Design review of the part shown in the three views and the two pictorial views. Dimensions are in mm from the part's minimum x, y and z. Coordinates: 2 decimals unless noted, no trailing zeros. Write each loop counter-clockwise with the first axis right and the second up, starting at its lowest first coordinate (ties: lowest second). Pieces come first, ordered by that corner, then holes. Notation, with made-up numbers: M -4.75,-28.75 L 5.25,-28.75 A13 cw 5.25,-14.75 Z; hole C 41.5,-19.5 d7. An arc over 180 degrees is marked long. One line per question, with ' | ' between items.
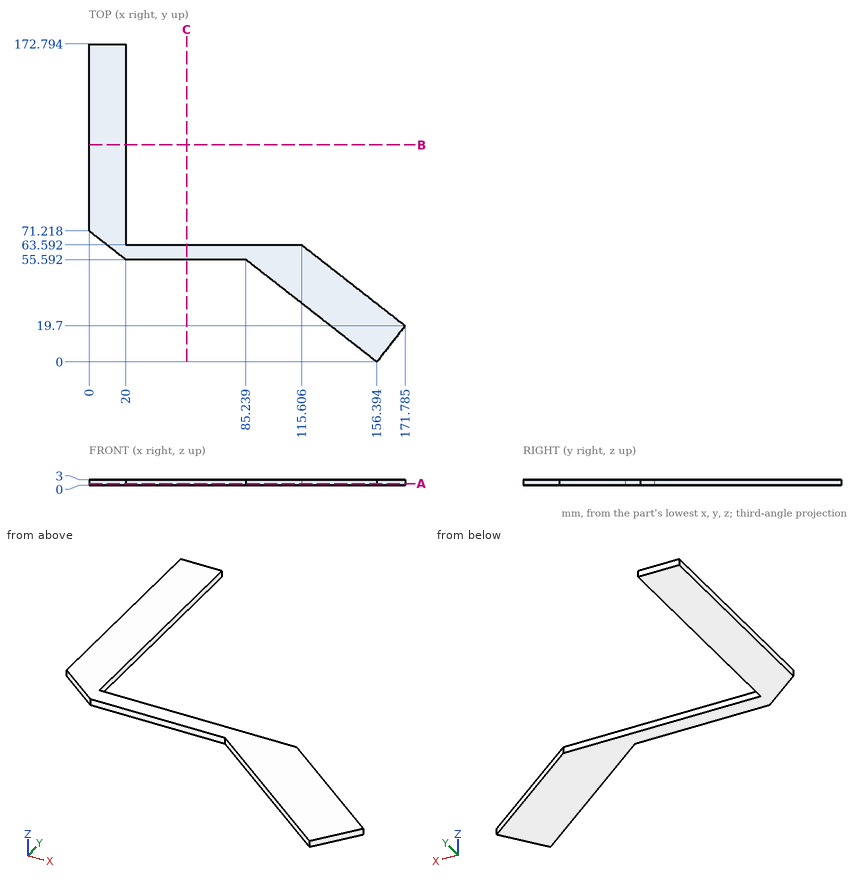
1. Take a section at C-C on x = 53. State the section outline as (y, z) points.
Computed values:
outline: M 55.59,0 L 63.59,0 L 63.59,3 L 55.59,3 Z
2. Take a section at B-B on y = 118. State the section outline as (x, z) points, plus the area to 3 significant figures.
Computed values:
outline: M 0,0 L 20,0 L 20,3 L 0,3 Z | area: 60.0 mm2
3. Clearance check with flat-ended pins moving along their axes: P1, Ø1.5, axis at y = 138, z = 2.5, coming from the -X side; P2, Ø0.9, axis at y = 123.5, z = 1, coming from the +X side; P3, Ø0.9, axis at x = 90, z = 2, coming from the +Y side; P4, Ø0.9, axis at x = 60.5, z = 2, coming from the -Y side. State where each tip first meets the part, or that it passes through.
Computed values:
P1: stops at x = 0 | P2: stops at x = 20 | P3: stops at y = 63.59 | P4: stops at y = 55.59
4. Take a section at A-A on z = 1. State the section outline as (x, y) points (1 decimal), plus the area to 3 significant figures.
Computed values:
outline: M 0,71.2 L 20,55.6 L 85.2,55.6 L 156.4,0 L 171.8,19.7 L 115.6,63.6 L 20,63.6 L 20,172.8 L 0,172.8 Z | area: 4,850 mm2
5. For line 1 along Y through (x, z) = (22, 1.05); line 2 along X through (y, z) = (130.5, 0.5); line 3 along X through (y, z) = (31, 1.55) (1 decimal), list the stretches that pass through material, from the lowest coordinate up.
Computed values:
line 1: y = 55.59 to 63.59 | line 2: x = 0 to 20 | line 3: x = 116.7 to 157.3
